For this review, use the dimensioned drawing (mm, ordinates from the lowest corner) and the shaded views. A direction names the side the tool comes from. Coordinates: 2 decimals unless noted, no trailing zeros. Write each loop counter-clockwise with the first axis right and the second up, starting at its lowest first coordinate (ties: lowest second). Pieces come first, ordered by that corner, then holes. Notation, with made-up numbers: (40, 0) -> (75, 0) arc R21 cw to (75, 12) -> close; hole circle Ø6 at (80.5, -24.75). An arc over 180 degrees is marked (long way). Put each result on its own line as item: value. Start each with the question number.
Item 1: Consider section D-D on y = 23. Give the boundary of the cut face in (x, z).
Item 2: Consider section C-C on y = 53.5. Give the boundary of the cut face in (x, z) (3 decimals).
Item 3: Consider section A-A on x = 67. Give the boundary of the cut face in (y, z) (3 decimals).
Item 4: Insertion check: P1, Ø3, axis at y = 25, z = 4, coming from the +X side; P2, Ø3, axis at x = 18, z = 1.5, coming from the +Y side; P3, Ø3.5, axis at x = 67, y = 53.5, coming from the +Z side; P4, Ø1.8, axis at x = 66.5, z = 1.5, coming from the +Y side. Each pin has a flat end and moves straight along its axis. Give the tip position at first contact, or say it passes through.
Item 5: To check wall thickness, follow L1, parallel to Y at x = 67, z = 1.95 (3 decimals); L2, parallel to Y at x = 67, z = 3.75; L3, parallel to Y at x = 14, z = 4.65. State the ranges of each line that lie inside material, in increasing order.
Item 6: Consider section B-B on z = 3.95. Give the boundary of the cut face in (x, y), and give its area (3 significant figures).
Item 7: For the marked faces 1, 2, 3, 4 and 5, list the 3-axis set-ups (+Z, -Z, +X, -X, +Y, -Y) from which the entire face can be reached by the end or side of a thin tool; tool diameter is ignored.
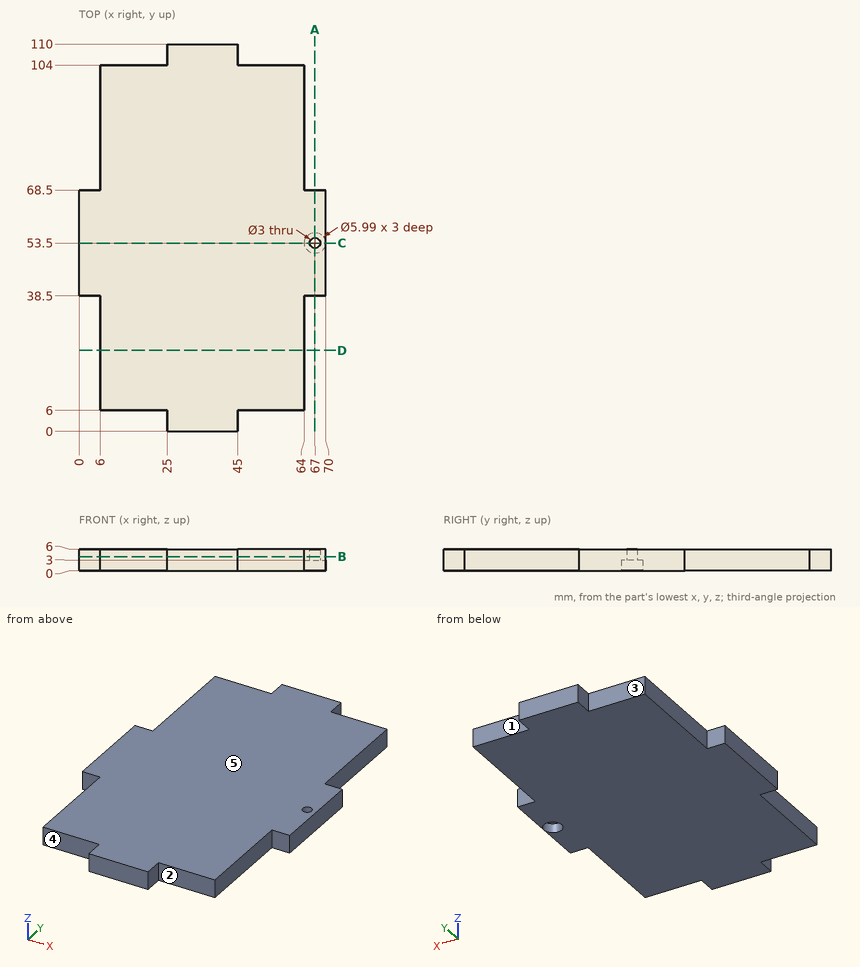
Return value:
1. outline: (6, 0) -> (64, 0) -> (64, 6) -> (6, 6) -> close
2. outline: (0, 0) -> (64.005, 0) -> (64.005, 3) -> (65.5, 3) -> (65.5, 6) -> (0, 6) -> close; (68.5, 3) -> (69.995, 3) -> (69.995, 0) -> (70, 0) -> (70, 6) -> (68.5, 6) -> close
3. outline: (38.5, 0) -> (50.505, 0) -> (50.505, 3) -> (52, 3) -> (52, 6) -> (38.5, 6) -> close; (55, 3) -> (56.495, 3) -> (56.495, 0) -> (68.5, 0) -> (68.5, 6) -> (55, 6) -> close
4. P1: x = 64
4. P2: y = 104
4. P3: z = 6
4. P4: y = 68.5
5. L1: 38.5 to 50.505, 56.495 to 68.5
5. L2: 38.5 to 52, 55 to 68.5
5. L3: 6 to 104
6. outline: (0, 38.5) -> (6, 38.5) -> (6, 6) -> (25, 6) -> (25, 0) -> (45, 0) -> (45, 6) -> (64, 6) -> (64, 38.5) -> (70, 38.5) -> (70, 68.5) -> (64, 68.5) -> (64, 104) -> (45, 104) -> (45, 110) -> (25, 110) -> (25, 104) -> (6, 104) -> (6, 68.5) -> (0, 68.5) -> close; hole circle Ø3 at (67, 53.5)
6. area: 6,280 mm^2
7. face 1: +Z, -Z, +X, +Y
7. face 2: +Z, -Z, +X, -Y
7. face 3: +Z, -Z, -X, +Y
7. face 4: +Z, -Z, -X, -Y
7. face 5: +Z, +X, -X, +Y, -Y
